Part model, mm, in its own coordinate system. Face numbers are marked on the shaded views. Give positions to 0.01 mm unless a question says otherwise; leave off trailing zeros. Answer as CSV lines item,"result". Start each with the question number.
Item 1: Two-plate mould, pull along Y, no slides. Class the marked faces 1 and 2: +Y half, -Y half, draft (parallel to the pull), parting line (faces both ways), or undercut.
Item 2: Band-saw the part on A-A, the plane y = 31.5. Count the separate pieces of the cut face and the enclosed holes in it, then the cut area to 3 significant figures.
Item 3: Pin check, flat tips, straight feed: pin 1 (3 mm diameter, centred on x = 35.5, z = 107, fed in from +Y); pin 2 (3 mm diameter, centred on x = 160, z = 95, fed in from -Y). Stop position of each tip, or through.
Item 4: Wall check: L1, parallel to Z at x = 198.35, y = 20; L2, parallel to Z at x = 40, y = 6; L3, parallel to X at y = 3.5, z = 230. Give the ranges that are in metal, low to high. Write a range as from..to.
from build123d import *

# Parameters (mm, degrees)
EXTRUDE_1_DEPTH       = 245
EXTRUDE_3_DEPTH       = 245
PATTERN_CURVE_1_COUNT = 19
PATTERN_CURVE_1_PITCH = 9.75
SKETCH_7_R            = 2.6
CUT_EXTRUDE_4_DEPTH   = 6
CUT_EXTRUDE_START     = -8
SKETCH_13_R           = 2.6
CUT_EXTRUDE_9_DEPTH   = 8
SKETCH_15_R           = 2.1
SKETCH_15_R_2         = 1.6
CUT_EXTRUDE_10_DEPTH  = 10


with BuildPart() as part:
    # Эскиз1 → Вытянуть1 (new body)
    with BuildSketch(Plane.XY):
        with BuildLine():
            Line((0, 45), (2.564446908, 45))
            ThreePointArc((2.564446908, 45), (3.247630994, 44.730246195), (3.562232066, 44.066519011))
            Line((3.562232066, 44.066519011), (5.5, 15))
            Line((5.5, 15), (194.5, 15))
            Line((194.5, 15), (196.437767934, 44.066519011))
            ThreePointArc((196.437767934, 44.066519011), (196.752369006, 44.730246195), (197.435553092, 45))
            Line((197.435553092, 45), (200, 45))
            Line((200, 45), (200, 0))
            Line((200, 0), (0, 0))
            Line((0, 0), (0, 45))
        make_face()
    extrude(amount=EXTRUDE_1_DEPTH)

    # Эскиз2 → Вытянуть3 (add)
    with BuildSketch(Plane.XY.offset(245)):
        with BuildLine():
            Line((11.5, 44.5), (10, 15))
            Line((10, 15), (14, 15))
            Line((14, 15), (12.5, 44.5))
            ThreePointArc((12.5, 44.5), (12, 45), (11.5, 44.5))
        make_face()
    extrude_3 = extrude(amount=-EXTRUDE_3_DEPTH)

    # Кривая1: Вытянуть3 ×19
    with Locations(*[(i * PATTERN_CURVE_1_PITCH, 0, 0) for i in range(1, PATTERN_CURVE_1_COUNT)]):
        add(extrude_3)

    # Эскиз7 → Вырез-Вытянуть4 (cut)
    with BuildSketch(Plane.ZY):
        with Locations(Location((22.5, 20, 0), (0, 0, 270))):
            Circle(SKETCH_7_R)
        with Locations(Location((222.5, 20, 0), (0, 0, 270))):
            Circle(SKETCH_7_R)
        with Locations(Location((122.5, 20, 0), (0, 0, 270))):
            Circle(SKETCH_7_R)
    extrude(amount=-CUT_EXTRUDE_4_DEPTH, mode=Mode.SUBTRACT)

    # Эскиз13 → Вырез-Вытянуть9 (cut)
    with BuildSketch(Plane(origin=(200, 0, 0), x_dir=(0, 0, -1), z_dir=(1, 0, 0)).offset(CUT_EXTRUDE_START)):
        with Locations(Location((-222.5, 20, 0), (0, 0, 270))):
            Circle(SKETCH_13_R)
        with Locations(Location((-122.5, 20, 0), (0, 0, 270))):
            Circle(SKETCH_13_R)
        with Locations(Location((-22.5, 20, 0), (0, 0, 270))):
            Circle(SKETCH_13_R)
    extrude(amount=CUT_EXTRUDE_9_DEPTH, mode=Mode.SUBTRACT)

    # Эскиз15 → Вырез-Вытянуть10 (cut)
    with BuildSketch(Plane.XZ):
        with Locations((45, 42)):
            Circle(SKETCH_15_R)
        with Locations((116.5, 142.4)):
            Circle(SKETCH_15_R_2)
        with Locations((83, 142.4)):
            Circle(SKETCH_15_R_2)
        with Locations((40, 230)):
            Circle(SKETCH_15_R_2)
        with Locations((160, 230)):
            Circle(SKETCH_15_R_2)
        with Locations((40, 95)):
            Circle(SKETCH_15_R_2)
        with Locations((160, 95)):
            Circle(SKETCH_15_R_2)
    extrude(amount=-CUT_EXTRUDE_10_DEPTH, mode=Mode.SUBTRACT)


solid = part.part
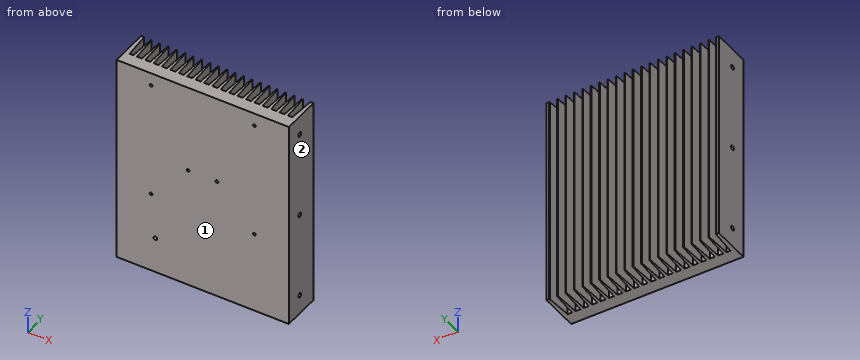
Output:
1,face 1,"-Y half"
1,face 2,"draft"
2,separate pieces,"21"
2,enclosed holes,"0"
2,area,"13,000 mm²"
3,pin 1,"y = 15"
3,pin 2,"y = 10"
4,L1,"0..19.9, 25.1..119.9, 125.1..219.9, 225.1..245"
4,L2,"0..93.4, 96.6..228.4, 231.6..245"
4,L3,"0..38.4, 41.6..158.4, 161.6..200"
